Design review of the part built by this model. Coordinates are the model's own, in mm. A direction names the side the tool comes from. Give positions to 0.01 mm unless a question says otherwise; leave off trailing zeros. Loops run counter-clockwise (first coordinate to the right, second up) from the corner with the lowest first, then second, coordinate; pieces in that order, holes last. Notation, with made-up numbers: (-8.75, 84.25) -> (45.25, 84.25) arc R5 ccw to (45.25, 89.25) -> close; hole circle Ø4 at (21.5, 80). An arc over 180 degrees is marked (long way). Use CSV: the item, a comma, the result in double quotes. Start each with the question number.
Item 1: We need section A-A (z = -6). State the section outline as (x, y) points.
Item 2: For faces 1 (the face through (12, -11, 0)), 2 (the face through (12, -30.5, -7)), list the 3-axis set-ups (+Z, -Z, +X, -X, +Y, -Y) from which the entire face can be reached by the end or side of a thin tool; tool diameter is ignored.
Item 3: The part is to be moulded in two halves that separate along X. For faces 3 (the face through (25.65, -28.98, -13.99)), 4 (the face through (24.298, -21.963, 1.479)), 5 (the face through (12.5, -26.5, -1)), say which applies: +X half, -X half, draft (parallel to the pull), parting line (faces both ways), or undercut.
Item 4: We need section D-D (x = 16.5). State the section outline as (y, z) points, plus the area to 4 significant figures.
Item 5: Wall thickness on line 1 along X through (y, z) = (-29.05, -7); line 2 along Y through (x, z) = (24.5, 1.4); line 3 along Z through (x, y) = (24.5, -7): over which ranges is each line inside the solid? List them lowest first. Write a range as from..to.
Item 6: Clearance check with flat-ended pins moving along their axes: pin 1 (7.5 mm diameter, centred on x = 11, z = -12, fed in from +Y); pin 2 (4 mm diameter, centred on x = 0, y = -23.5, fed in from +Z); pin 3 (1.5 mm diameter, centred on x = 24, y = -15, fed in from -Z); pin 4 (5 mm diameter, centred on x = 24.5, y = -23.5, fed in from -Z). State where each tip first meets the part, or that it passes through.
Item 7: We need section B-B (y = -23.5). State the section outline as (x, z) points.
Item 8: We need section C-C (z = 1). State the section outline as (x, y) points.
from build123d import *

# Parameters (mm, degrees)
SKETCH_1_R          = 1.55
EXTRUDE_1_DEPTH     = 3
SKETCH_2_W          = 32.5
SKETCH_2_H          = 3
EXTRUDE_2_DEPTH     = 17
SKETCH_3_R          = 2.6
CUT_EXTRUDE_1_DEPTH = 17
CHAMFER_1_SIZE      = 2
FILLET_1_R          = 10
FILLET_2_R          = 5


with BuildPart() as part:
    # 草图1 → 凸台-拉伸1 (new body)
    with BuildSketch(Plane.XY):
        Polygon((28.5, -27.5), (28.5, -30.5), (-4, -30.5), (-4, -27.5), (-4, 4), (28.5, 4), align=None)
        Circle(SKETCH_1_R, mode=Mode.SUBTRACT)
        with Locations((24.5, 0)):
            Circle(SKETCH_1_R, mode=Mode.SUBTRACT)
        with Locations((0, -23.5)):
            Circle(SKETCH_1_R, mode=Mode.SUBTRACT)
        with Locations((24.5, -23.5)):
            Circle(SKETCH_1_R, mode=Mode.SUBTRACT)
    extrude(amount=EXTRUDE_1_DEPTH)

    # 草图2 → 凸台-拉伸2 (add)
    with BuildSketch(Plane(origin=(0, 0, 0), x_dir=(-1, 0, 0), z_dir=(0, 0, -1))):
        with Locations((-12.25, -29)):
            Rectangle(SKETCH_2_W, SKETCH_2_H)
    extrude(amount=EXTRUDE_2_DEPTH)

    # 草图3 → 切除-拉伸1 (cut)
    with BuildSketch(Plane.XZ.offset(30.5)):
        with Locations(Location((22.25, -7, 0), (0, 0, 270))):
            Circle(SKETCH_3_R)
        with Locations(Location((2.25, -7, 0), (0, 0, 270))):
            Circle(SKETCH_3_R)
    extrude(amount=-CUT_EXTRUDE_1_DEPTH, mode=Mode.SUBTRACT)

    # 倒角1
    chamfer_1_edges = [part.edges().sort_by_distance(p)[0] for p in [
        (12.25, -27.5, 0),
    ]]
    chamfer(chamfer_1_edges, length=CHAMFER_1_SIZE)

    # 圆角1
    fillet_1_edges = [part.edges().sort_by_distance(p)[0] for p in [
        (28.5, -29, -17),
        (-4, -29, -17),
    ]]
    fillet(fillet_1_edges, radius=FILLET_1_R)

    # 圆角2
    fillet_2_edges = [part.edges().sort_by_distance(p)[0] for p in [
        (-4, 4, 1.5),
        (28.5, 4, 1.5),
    ]]
    fillet(fillet_2_edges, radius=FILLET_2_R)


solid = part.part
Results found:
1,outline,"(-4, -30.5) -> (-0.15, -30.5) -> (-0.15, -27.5) -> (-4, -27.5) -> close; (4.65, -30.5) -> (19.85, -30.5) -> (19.85, -27.5) -> (4.65, -27.5) -> close; (24.65, -30.5) -> (28.5, -30.5) -> (28.5, -27.5) -> (24.65, -27.5) -> close"
2,face 1,"-Z, +X, -X, +Y"
2,face 2,"+Z, -Z, +X, -X, -Y"
3,face 3,"+X half"
3,face 4,"undercut"
3,face 5,"draft"
4,outline,"(-30.5, -17) -> (-27.5, -17) -> (-27.5, -2) -> (-25.5, 0) -> (4, 0) -> (4, 3) -> (-30.5, 3) -> close"
4,area,"156.5 mm²"
5,line 1,"-4..-0.35, 4.85..19.65, 24.85..28.5"
5,line 2,"-30.5..-25.05, -21.95..-1.55, 1.55..3.9"
5,line 3,"0..3"
6,pin 1,"y = -27.5"
6,pin 2,"z = 3"
6,pin 3,"z = 0"
6,pin 4,"z = -0.5"
7,outline,"(-4, 0) -> (-1.55, 0) -> (-1.55, 3) -> (-4, 3) -> close; (1.55, 0) -> (22.95, 0) -> (22.95, 3) -> (1.55, 3) -> close; (26.05, 0) -> (28.5, 0) -> (28.5, 3) -> (26.05, 3) -> close"
8,outline,"(-4, -30.5) -> (28.5, -30.5) -> (28.5, -1) arc R5 ccw to (23.5, 4) -> (1, 4) arc R5 ccw to (-4, -1) -> close; hole circle Ø3.1 at (0, -23.5); hole circle Ø3.1 at (0, 0); hole circle Ø3.1 at (24.5, -23.5); hole circle Ø3.1 at (24.5, 0)"
